For this review, take the finished solid that the model builds, in its own axes (mm). A direction names the side the tool comes from. Round coordinates to 2 decimals unless told otherwise and drop trailing zeros. Write each loop counter-clockwise with the first axis right and the second up, starting at its lowest first coordinate (ties: lowest second). Pieces come first, ordered by that corner, then holes. Notation, with made-up numbers: (-28.5, 26) - (6.5, 26) arc R20 cw to (6.5, 51) - close; hole circle Ø5 at (45.25, 60.5). An arc over 180 degrees is marked (long way). Answer in a Markdown table with one row per item. Add a question column.
from build123d import *

# Parameters (mm, degrees)
F0_W     = 127
F0_H     = 76.2
F1_DEPTH = 50.8
F2_R     = 12.7
F3_DEPTH = 38.1
F4_R     = 12.7
F5_DEPTH = 76.2


with BuildPart() as f1:
    # F0 (on Front) → F1 (new body)
    with BuildSketch(Plane.XZ):
        Rectangle(F0_W, F0_H)
    extrude(amount=F1_DEPTH)

    # F2 (on face) → F3 (cut)
    with BuildSketch(Plane.XZ.offset(50.8)):
        Circle(F2_R)
    extrude(amount=-F3_DEPTH, mode=Mode.SUBTRACT)

    # F4 (on face) → F5 (cut)
    with BuildSketch(Plane(origin=(-63.5, 0, 0), x_dir=(0, -1, 0), z_dir=(-1, 0, 0))):
        with Locations((25.4, 0)):
            Circle(F4_R)
    extrude(amount=-F5_DEPTH, mode=Mode.SUBTRACT)


solid = f1.part
Q1. Add section A-A on z = 6.5. State the section outline as (x, y) points.
Q2. To check wall thickness, follow probe 1 along Z at (x, y) = (-28.5, -25.4); probe 2 along X at (y, z) = (-43.5, -6); probe 3 along X at (y, z) = (-35, 0). State the ranges of each line that lie inside material, in increasing order.
Q3. Insertion check: pin 1 Ø12.5 at (x, z) = (0.5, 3) entering from -Y; pin 2 Ø23 at (y, z) = (-25.4, 0) entering from -X. Each pin has a flat end and moves straight along its axis. Give the tip position at first contact, or say it passes through.
Q4. Add section B-B on x = -20. State the section outline as (y, z) points, then the cut area to 3 significant figures.
Q5. Add section C-C on y = -18.5. State the section outline as (x, z) points, then the cut area to 3 significant figures.
Q6. Tool access review of faces 1 (the face through (8.2, -25.5, 12.7)), 2 (the face through (13, -50.8, 1)), 3 (the face through (0, -12.7, 0)): name each direction out of +Z, -Z, +X, -X, +Y, -Y from which nothing blocks a thin tool from reaching the whole face with its end or side.
Q7. Draft analysis for pull direction X (two halves, no side actions). For faces 4 (the face through (12.7, -25, 0)), 5 (the face through (6.827, -41.1, 10.709)), 6 (the face through (-1, -25, 38.1)), state which applies: released by +X, released by -X, zero draft, split by the parting line, or undercut.
Answer sheet:
| question | item | result |
|---|---|---|
| 1 | outline | (-63.5, -50.8) - (-10.91, -50.8) - (-10.91, -36.31) - (-63.5, -36.31) - close; (-63.5, -14.49) - (-10.91, -14.49) - (-10.91, -12.7) - (10.91, -12.7) - (10.91, -14.49) - (12.7, -14.49) - (12.7, -36.31) - (10.91, -36.31) - (10.91, -50.8) - (63.5, -50.8) - (63.5, 0) - (-63.5, 0) - close |
| 2 | probe 1 | z = -38.1 to -12.7, 12.7 to 38.1 |
| 2 | probe 2 | x = -63.5 to -11.19, 11.19 to 63.5 |
| 2 | probe 3 | x = 12.7 to 63.5 |
| 3 | pin 1 | stops at y = -12.7 |
| 3 | pin 2 | stops at x = 12.7 |
| 4 | outline | (-50.8, -38.1) - (0, -38.1) - (0, 38.1) - (-50.8, 38.1) - close; hole circle Ø25.4 at (-25.4, 0) |
| 4 | area | 3,360 mm² |
| 5 | outline | (-63.5, -38.1) - (63.5, -38.1) - (63.5, 38.1) - (-63.5, 38.1) - (-63.5, 10.66) - (-6.9, 10.66) arc R12.7 cw to (6.9, 10.66) - (12.7, 10.66) - (12.7, -10.66) - (6.9, -10.66) arc R12.7 cw to (-6.9, -10.66) - (-63.5, -10.66) - close |
| 5 | area | 8,010 mm² |
| 6 | face 1 | -X |
| 6 | face 2 | +Z, -Z, +X, -X, -Y |
| 6 | face 3 | -Y |
| 7 | face 4 | released by -X |
| 7 | face 5 | undercut |
| 7 | face 6 | zero draft |
